Build history of the part. All positions in model axes, mm. A direction names the side the tool comes from. Round coordinates to 2 decimals unless told otherwise and drop trailing zeros. Use one line per item in the form item = value. Start each with the question number.
Q1. 3-axis set-ups, long thin cutter, end or side, ignore diameter. For faces 4 (the face through (-56.7, 24.92, -24.42)), 5 (the face through (-12.7, 13, -24)): which of +Z, -Z, +X, -X, +Y, -Y reach the whole face in a straight line?
Q2. Mould opens along Z. For faces 1 (the face through (-6, 18.258, -8)), 2 (the face through (-28.2, 0.9, -47.3)), 3 (the face through (0, 5, -24)) say: released by +Z, released by -Z, zero draft, split by the parting line, or undercut.
Q3. Drill centre lines: line 1 (Y direction, x = -10, z = -24); line 2 (X direction, y = 5.75, z = -2); line 3 (X direction, y = 11.25, z = -33). Where is each one in solid material? Low to high.
Q4. Pin check, flat tip, straight feed: pin 1 (6 mm diameter, centred on y = 22.5, z = -7, fed in from -X). Stop position of the tip, or through.
Autodesk Inventor part; units mm, degrees
ref_plane "YZ Plane" through (0, 0, 0) normal (1, 0, 0) x (0, 1, 0)
ref_plane "XZ Plane" through (0, 0, 0) normal (0, 1, 0) x (-1, 0, 0)
ref_plane "XY Plane" through (0, 0, 0) normal (0, 0, 1) x (1, 0, 0)
sketch "Sketch1" plane through (0, 0, 0) normal (0, 1, 0) x (-1, 0, 0)
  line L0 (0, 0) -> (57.15, 0)
  line L1 (57.15, 0) -> (57.15, -48.26)
  line L2 (57.15, -48.26) -> (0, -48.26)
  line L3 (0, -48.26) -> (0, 0)
  dimension "d0" = 57.15
  dimension "d1" = 48.26
extrude "Extrusion1" add sketch "Sketch1" along normal blind 25.4
sketch "Sketch2" plane through (0, 0, 0) normal (1, 0, 0) x (0, 0, -1)
  line L0 (0, 0) -> (48.26, 0) construction
  line L1 (48.26, 0) -> (48.26, 25.4) construction
  line L2 (0, 25.4) -> (48.26, 25.4) construction
  line L3 (0, 0) -> (0, 25.4) construction
  line L4 (14.8042, 6.663) -> (33.4558, 6.663)
  line L5 (33.4558, 6.663) -> (33.4558, 18.737)
  line L6 (33.4558, 18.737) -> (14.8042, 18.737)
  line L7 (14.8042, 18.737) -> (14.8042, 6.663)
  line L8 (14.8042, 6.663) -> (33.4558, 18.737) construction
  line L9 (33.4558, 6.663) -> (14.8042, 18.737) construction
  line L10 (4.1311, 15.5562) -> (11.3642, 15.5562)
  line L11 (11.3642, 15.5562) -> (11.3642, 18.2577)
  line L12 (11.3642, 18.2577) -> (4.1311, 18.2577)
  line L13 (4.1311, 18.2577) -> (4.1311, 15.5562)
  line L14 (4.1311, 15.5562) -> (11.3642, 18.2577) construction
  line L15 (11.3642, 15.5562) -> (4.1311, 18.2577) construction
  point P0 (24.13, 12.7)
  point P1 (7.7477, 16.9069)
extrude "Extrusion2" cut sketch "Sketch2" against normal blind 12.7
sketch "Sketch3" plane through (-57.15, 0, -48.26) normal (-1, 0, 0) x (0, 0, 1)
  line L0 (0, 0) -> (48.26, 0)
  line L1 (48.26, 0) -> (48.26, 25.4)
  line L2 (0, 25.4) -> (48.26, 25.4)
  line L3 (0, 0) -> (0, 25.4)
  circle A0 centre (24.13, 12.7) radius 2.54
  dimension "d6" = 5.08
extrude "Extrusion3" add sketch "Sketch3" along normal blind 7.62 contours A0
chamfer "Chamfer1" distance 0.254 distance2 7.62 1 edges at (-64.77, 12.7, -26.67) measured on face at (-64.77, 13.2614, -23.2922)
fillet "Fillet1" radius 3.175 4 edges at (-28.575, 25.4, -48.26) (-28.575, 0, -48.26) (-28.575, 0, 0) (-28.575, 25.4, 0)
fillet "Fillet2" radius 1.5875 18 edges at (0, 24.4701, -47.3301) (0, 12.7, -48.26) (0, 0.9299, -47.3301) (0, 0, -24.13) (0, 0.9299, -0.9299) (0, 12.7, 0) (0, 24.4701, -0.9299) (0, 25.4, -24.13) (-57.15, 24.4701, -0.9299) (-57.15, 12.7, 0) (-57.15, 0.9299, -0.9299) (-57.15, 0, -24.13) (-57.15, 0.9299, -47.3301) (-57.15, 12.7, -48.26) (-57.15, 24.4701, -47.3301) (-57.15, 25.4, -24.13) (-57.15, 12.7, -26.67) (-57.1505, 12.7, -26.67)
properties part number "PoEbox"
Report:
q1.face_4 = +Z, -Z, -X, +Y
q1.face_5 = +X
q2.face_1 = undercut
q2.face_2 = released by -Z
q2.face_3 = zero draft
q3.line_1 = 0 to 6.66, 18.74 to 25.4
q3.line_2 = -57.15 to 0
q3.line_3 = -57.15 to -12.7
q4.pin_1 = -57.15
